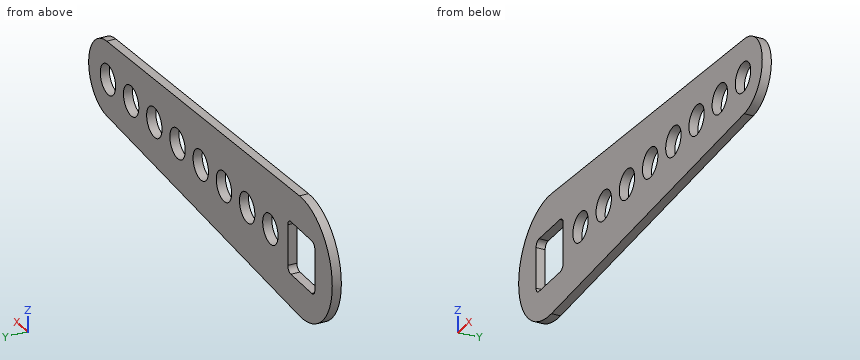
```python
from build123d import *

# Parameters (mm, degrees)
SKETCH1_R           = 3.96875
BOSS_EXTRUDE1_DEPTH = 2.4


with BuildPart() as part:
    # Sketch1 → Boss-Extrude1 (new body)
    with BuildSketch(Plane(origin=(0, 0, 0), x_dir=(1, 0, 0), z_dir=(0, 1, 0))):
        with BuildLine():
            Line((0.965, 15.970872706), (100.601240234, 9.950602331))
            ThreePointArc((100.601240234, 9.950602331), (109.96875, 0), (100.601240234, -9.950602331))
            Line((100.601240234, -9.950602331), (0.965, -15.970872706))
            ThreePointArc((0.965, -15.970872706), (-16, 0), (0.965, 15.970872706))
        make_face()
        with Locations((16, 0)):
            Circle(SKETCH1_R, mode=Mode.SUBTRACT)
        with Locations((28, 0)):
            Circle(SKETCH1_R, mode=Mode.SUBTRACT)
        with Locations((40, 0)):
            Circle(SKETCH1_R, mode=Mode.SUBTRACT)
        with Locations((52, 0)):
            Circle(SKETCH1_R, mode=Mode.SUBTRACT)
        with Locations((64, 0)):
            Circle(SKETCH1_R, mode=Mode.SUBTRACT)
        with Locations((76, 0)):
            Circle(SKETCH1_R, mode=Mode.SUBTRACT)
        with Locations((88, 0)):
            Circle(SKETCH1_R, mode=Mode.SUBTRACT)
        with Locations((100, 0)):
            Circle(SKETCH1_R, mode=Mode.SUBTRACT)
        with BuildLine():
            Line((-5.4, 7), (5.4, 7))
            ThreePointArc((5.4, 7), (6.53137085, 6.53137085), (7, 5.4))
            Line((7, 5.4), (7, -5.4))
            ThreePointArc((7, -5.4), (6.53137085, -6.53137085), (5.4, -7))
            Line((5.4, -7), (-5.4, -7))
            ThreePointArc((-5.4, -7), (-6.53137085, -6.53137085), (-7, -5.4))
            Line((-7, -5.4), (-7, 5.4))
            ThreePointArc((-7, 5.4), (-6.53137085, 6.53137085), (-5.4, 7))
        make_face(mode=Mode.SUBTRACT)
    extrude(amount=BOSS_EXTRUDE1_DEPTH)


solid = part.part
```
Can you work these out from the model? Positions are in its coordinate system, mm. Round coordinates to 2 decimals unless told otherwise and drop trailing zeros. Loops run counter-clockwise (first coordinate to the right, second up) from the corner with the lowest first, then second, coordinate; pieces in that order, holes last. Notation, with made-up numbers: (50.25, -37) -> (74.25, -37) arc R24 cw to (74.25, -10) -> close; hole circle Ø8 at (41.5, 61.5). An arc over 180 degrees is marked (long way). Answer in a Markdown table with one row per item.
Item 1: Suppose I cut it at C-C, the plane x = 52. List the corners of the cut face in (y, z) for me, plus the area to 3 significant figures.
Answer block:
| item | result |
|---|---|
| outline | (0, -12.89) -> (2.4, -12.89) -> (2.4, -3.97) -> (0, -3.97) -> close; (0, 3.97) -> (2.4, 3.97) -> (2.4, 12.89) -> (0, 12.89) -> close |
| area | 42.8 mm² |
Item 2: Will these pins go through, and if not, where does the flat tip stop? P1, Ø1, axis at x = 72, y = 1, coming from the +Z side; P2, Ø6.5, axis at x = 88, z = 0, coming from the -Y side; P3, Ø1.2, axis at x = -2.5, y = 2, coming from the -Z side.
Answer block:
| item | result |
|---|---|
| P1 | z = 11.71 |
| P2 | through |
| P3 | z = -15.89 |
Item 3: Suppose I cut it at B-B, the plane x = 88. List the corners of the cut face in (y, z) for me, plus the area to 3 significant figures.
Answer block:
| item | result |
|---|---|
| outline | (0, -10.71) -> (2.4, -10.71) -> (2.4, -3.97) -> (0, -3.97) -> close; (0, 3.97) -> (2.4, 3.97) -> (2.4, 10.71) -> (0, 10.71) -> close |
| area | 32.4 mm² |
Item 4: If I drill on probe 1 along Z at (x, y) = (3.5, 1.7); probe 2 along Z at (x, y) = (51, 0.65); probe 3 along X at (y, z) = (1.8, -6.5), over which ranges is the centre line in solid material (lowest first)?
Answer block:
| item | result |
|---|---|
| probe 1 | -15.82 to -7, 7 to 15.82 |
| probe 2 | -12.95 to -3.84, 3.84 to 12.95 |
| probe 3 | -14.62 to -6.56, 6.56 to 107.56 |
Item 5: Suppose I cut it at A-A, the plane y = 0.9. Give the number of separate pieces and of enclosed holes in the cut face, plus the area to 3 significant figures.
Answer block:
| item | result |
|---|---|
| separate pieces | 1 |
| enclosed holes | 9 |
| area | 2,570 mm² |
